```python
from build123d import *

# Parameters (mm, degrees)
FILLET_1_R = 2


with BuildPart() as part:
    # 草图1 → 旋转1 (revolve)
    with BuildSketch(Plane.XY, mode=Mode.PRIVATE) as revolve_1_sk:
        Polygon((0, 0), (-2, 0), (-2, 8), (-5, 8), (-5, 3), (-7, 3), (-7, 8), (-10, 8), (-10, -2), (-75, -2), (-75, -22), (0, -22), align=None)
    revolve(revolve_1_sk.sketch.rotate(Axis((0, -198.175933826, 0), (0, 1, 0)), 180), axis=Axis((0, -198.175933826, 0), (0, 1, 0)))

    # 圆角1
    fillet_1_edges = [part.edges().sort_by_distance(p)[0] for p in [
        (-10, -2, 0),
    ]]
    fillet(fillet_1_edges, radius=FILLET_1_R)


solid = part.part
```
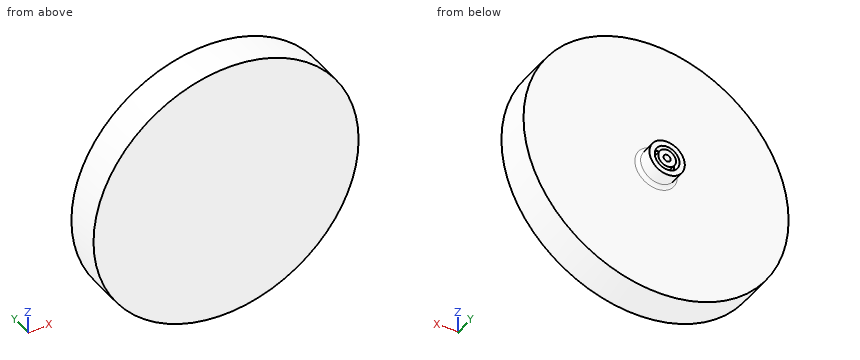
The model under review builds one solid part; all positions refer to its coordinate system, in mm. Coordinates: 2 decimals unless noted, no trailing zeros. Loops run counter-clockwise (first coordinate to the right, second up) from the corner with the lowest first, then second, coordinate; pieces in that order, holes last. Notation, with made-up numbers: (84.5, 61) -> (90.5, 61) arc R14 ccw to (90.5, 72) -> close; hole circle Ø7 at (89.5, -10). An arc over 180 degrees is marked (long way). Answer as CSV lines item,"result".
Item 1: Take a section at D-D, the plane x = 45. State the section outline as (y, z) points, and give its area (3 significant figures).
Results below:
outline,"(-22, -60) -> (-2, -60) -> (-2, 60) -> (-22, 60) -> close"
area,"2,400 mm2"
Item 2: Take a section at A-A, the plane x = 0. State the section outline as (y, z) points, and give its area (3 significant figures).
Results below:
outline,"(-22, -75) -> (-2, -75) -> (-2, -12) arc R2 cw to (0, -10) -> (8, -10) -> (8, -7) -> (3, -7) -> (3, -5) -> (8, -5) -> (8, -2) -> (0, -2) -> (0, 2) -> (8, 2) -> (8, 5) -> (3, 5) -> (3, 7) -> (8, 7) -> (8, 10) -> (0, 10) arc R2 cw to (-2, 12) -> (-2, 75) -> (-22, 75) -> close"
area,"3,150 mm2"
Item 3: Take a section at C-C, the plane y = -20. State the section outline as (x, z) points.
Results below:
outline,"circle Ø150 at (0, 0)"
Item 4: Insertion check: pin 1 (3 mm diameter, centred on x = 41.5, z = 7.5, fed in from +Y); pin 2 (3 mm diameter, centred on y = -11, z = -14.5, fed in from -X); pin 3 (2 mm diameter, centred on x = 0, z = -0.5, fed in from +Y). Each pin has a flat end and moves straight along its axis. Give the tip position at first contact, or say it passes through.
Results below:
pin 1,"stops at y = -2"
pin 2,"stops at x = -73.86"
pin 3,"stops at y = 0"
Item 5: Take a section at B-B, the plane z = 0. State the section outline as (x, y) points.
Results below:
outline,"(-75, -22) -> (75, -22) -> (75, -2) -> (12, -2) arc R2 cw to (10, 0) -> (10, 8) -> (7, 8) -> (7, 3) -> (5, 3) -> (5, 8) -> (2, 8) -> (2, 0) -> (-2, 0) -> (-2, 8) -> (-5, 8) -> (-5, 3) -> (-7, 3) -> (-7, 8) -> (-10, 8) -> (-10, 0) arc R2 cw to (-12, -2) -> (-75, -2) -> close"
Item 6: For L1, parallel to Z at x = 0, y = 5.5; L2, parallel to Z at x = 0, y = 2; L3, parallel to Y at x = 56, z = -32.5, list the stretches that pass through material, from the lowest coordinate up.
Results below:
L1,"z = -10 to -7, -5 to -2, 2 to 5, 7 to 10"
L2,"z = -10 to -2, 2 to 10"
L3,"y = -22 to -2"
